Autodesk Inventor part; units mm, degrees
ref_plane "YZ Plane" through (0, 0, 0) normal (1, 0, 0) x (0, 1, 0)
ref_plane "XZ Plane" through (0, 0, 0) normal (0, 1, 0) x (-1, 0, 0)
ref_plane "XY Plane" through (0, 0, 0) normal (0, 0, 1) x (1, 0, 0)
sketch "Sketch1" plane through (0, 0, 0) normal (0, 1, 0) x (-1, 0, 0)
  line L0 (6.35, -3.6662) -> (0, -7.3323)
  line L1 (0, -7.3323) -> (-6.35, -3.6662)
  line L2 (-6.35, -3.6662) -> (-6.35, 3.6662)
  line L3 (-6.35, 3.6662) -> (0, 7.3323)
  line L4 (0, 7.3323) -> (6.35, 3.6662)
  line L5 (6.35, 3.6662) -> (6.35, -3.6662)
  point P0 (0, 0)
  point P1 (0, 0)
  point P2 (0, 0)
  dimension "d0" = 12.7
extrude "Extrusion1" add sketch "Sketch1" along normal blind 497.5606
sketch "Sketch2" plane through (0, 0, 0) normal (0, -1, 0) x (1, 0, 0)
  point P0 (0, 0)
  point P1 (0, 0)
hole "Hole1" at (0, 0, 0) direction (0, 1, 0) diameter 4.9784 depth 25.4
sketch "Sketch3" plane through (0, 497.5606, 0) normal (0, 1, 0) x (1, 0, 0)
  point P0 (0, 0)
  point P1 (0, 0)
hole "Hole2" at (0, 497.5606, 0) direction (0, -1, 0) diameter 4.9784 depth 25.4
properties part number "Intake HexShaft 1" material "Aluminum 6061"
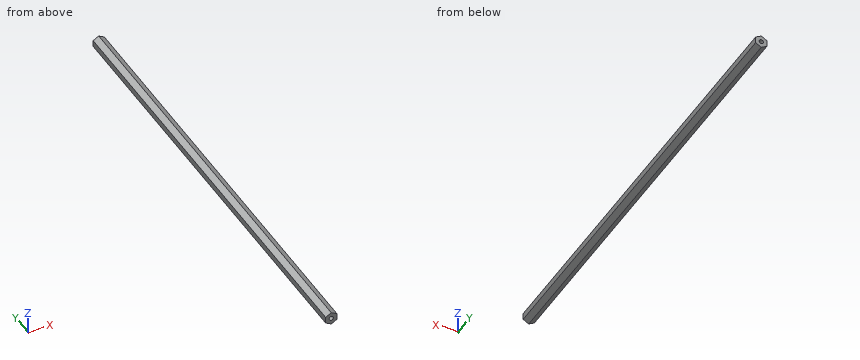
The listing builds one solid part. Answer for the finished solid, in the listing's coordinates (mm). Give positions to 0.01 mm unless a question says otherwise; leave off trailing zeros. Write each loop counter-clockwise with the first axis right and the second up, starting at its lowest first coordinate (ties: lowest second). Pieces come first, ordered by that corner, then holes.
Item 1: Flat-ended cylindrical pins translate along their axes: P1, Ø6, axis at x = -1, y = 346, coming from the +Z side; P2, Ø2.5, axis at x = 1, z = 0, coming from the +Y side; P3, Ø1, axis at x = -5, y = 229.5, coming from the -Z side. Find the tip coordinate at first contact, or state that the pin passes through.
Item 2: Find the intervals of material crossed by line 1 along Z through (x, y) = (0, 6.25); line 2 along X through (y, z) = (13.75, 0); line 3 along Y through (x, z) = (-1.5, 1), in increasing order.
Item 3: Section B-B, the plane z = 0 is taken. Write down the section's boundary in (x, y).
Item 4: Section A-A, the plane y = 73 is taken. Write down the section's boundary in (x, z).
Completed:
1. P1: stops at z = 7.33
1. P2: stops at y = 472.16
1. P3: stops at z = -4.73
2. line 1: z = -7.33 to -2.49, 2.49 to 7.33
2. line 2: x = -6.35 to -2.49, 2.49 to 6.35
2. line 3: y = 25.4 to 472.16
3. outline: (-6.35, 0) - (-2.49, 0) - (-2.49, 25.4) - (2.49, 25.4) - (2.49, 0) - (6.35, 0) - (6.35, 497.56) - (2.49, 497.56) - (2.49, 472.16) - (-2.49, 472.16) - (-2.49, 497.56) - (-6.35, 497.56) - close
4. outline: (-6.35, -3.67) - (0, -7.33) - (6.35, -3.67) - (6.35, 3.67) - (0, 7.33) - (-6.35, 3.67) - close
